from build123d import *

# Parameters (mm, degrees)
ESQUISSE1_W                  = 60
ESQUISSE1_H                  = 40
BOSS_EXTRU_1_DEPTH           = 6
ESQUISSE2_R                  = 1.75
ESQUISSE2_R_2                = 3.5
ENL_V_MAT_EXTRU_1_DEPTH      = 1
ENL_V_MAT_EXTRU_1_DEPTH_BACK = 7
CONG_1_R                     = 6


with BuildPart() as part:
    # Esquisse1 → Boss.-Extru.1 (new body)
    with BuildSketch(Plane.XY):
        with Locations((30, 20)):
            Rectangle(ESQUISSE1_W, ESQUISSE1_H)
    extrude(amount=BOSS_EXTRU_1_DEPTH)

    # Esquisse2 → Enlèv. mat.-Extru.1 (cut, two sides)
    with BuildSketch(Plane.XY.offset(6)) as enl_v_mat_extru_1_sk:
        with Locations((20, 30)):
            Circle(ESQUISSE2_R)
        with Locations((40, 30)):
            Circle(ESQUISSE2_R)
        with Locations((40, 10)):
            Circle(ESQUISSE2_R)
        with Locations((20, 10)):
            Circle(ESQUISSE2_R)
        with Locations((7.5, 20)):
            Circle(ESQUISSE2_R_2)
        with Locations((52.5, 20)):
            Circle(ESQUISSE2_R_2)
    extrude(amount=ENL_V_MAT_EXTRU_1_DEPTH, mode=Mode.SUBTRACT)
    extrude(enl_v_mat_extru_1_sk.sketch, amount=-ENL_V_MAT_EXTRU_1_DEPTH_BACK, mode=Mode.SUBTRACT)

    # Congé1
    cong_1_edges = [part.edges().sort_by_distance(p)[0] for p in [
        (0, 40, 3),
        (60, 40, 3),
        (60, 0, 3),
        (0, 0, 3),
    ]]
    fillet(cong_1_edges, radius=CONG_1_R)


solid = part.part
The listing builds one solid part. Answer for the finished solid, in the listing's coordinates (mm). Give positions to 0.01 mm unless a question says otherwise; leave off trailing zeros. Loops run counter-clockwise (first coordinate to the right, second up) from the corner with the lowest first, then second, coordinate; pieces in that order, holes last. Notation, with made-up numbers: M 5,42.25 L 20,42.25 A6 ccw 20,50.25 Z; hole C 87,59 d3. An arc over 180 degrees is marked long. Answer as CSV lines item,"result".
Item 1: The part is cut by section C-C (x = 40). Give the vertices of the cut face in (y, z), and give its area (3 significant figures).
Values follow:
outline,"M 0,0 L 8.25,0 L 8.25,6 L 0,6 Z; M 11.75,0 L 28.25,0 L 28.25,6 L 11.75,6 Z; M 31.75,0 L 40,0 L 40,6 L 31.75,6 Z"
area,"198 mm^2"
Item 2: The part is cut by section A-A (x = 52.5). Give the vertices of the cut face in (y, z), and give its area (3 significant figures).
Values follow:
outline,"M 0,0 L 16.5,0 L 16.5,6 L 0,6 Z; M 23.5,0 L 40,0 L 40,6 L 23.5,6 Z"
area,"198 mm^2"
Item 3: The part is cut by section D-D (z = 4.65). Give the vertices of the cut face in (x, y), and give its area (3 significant figures).
Values follow:
outline,"M 0,6 A6 ccw 6,0 L 54,0 A6 ccw 60,6 L 60,34 A6 ccw 54,40 L 6,40 A6 ccw 0,34 Z; hole C 7.5,20 d7; hole C 20,10 d3.5; hole C 20,30 d3.5; hole C 40,10 d3.5; hole C 40,30 d3.5; hole C 52.5,20 d7"
area,"2,250 mm^2"
Item 4: The mould has two halves that part along Y. Classify faces 1 (the flat face through (30, 40, 3)), 2 (the flat face through (0, 20, 3)), 3 (the cylindrical face through (18.25, 30.08, 3.04)): released by +Y, released by -Y, zero draft, split by the parting line, or undercut.
Values follow:
face 1,"released by +Y"
face 2,"zero draft"
face 3,"undercut"
Item 5: The part is cut by section B-B (y = 10). Give the vertices of the cut face in (x, z).
Values follow:
outline,"M 0,0 L 18.25,0 L 18.25,6 L 0,6 Z; M 21.75,0 L 38.25,0 L 38.25,6 L 21.75,6 Z; M 41.75,0 L 60,0 L 60,6 L 41.75,6 Z"
Item 6: Straight lines are drawn through the part: line 1 along Y through (x, z) = (19.5, 0.7); line 2 along X through (y, z) = (23, 5.3); line 3 along X through (y, z) = (9, 1). For each, find the intervals that lie inside material, in ascending order. Write a range as [from, to].
Values follow:
line 1,"y = [0, 8.32], [11.68, 28.32], [31.68, 40]"
line 2,"x = [0, 5.7], [9.3, 50.7], [54.3, 60]"
line 3,"x = [0, 18.56], [21.44, 38.56], [41.44, 60]"
